from build123d import *

# Parameters (mm, degrees)
CYLINDER_R     = 10
CYLINDER_DEPTH = 2
BOX_W          = 50
BOX_H          = 51
BOX_DEPTH      = 3
BOX001_W       = 50
BOX001_H       = 1
BOX001_DEPTH   = 25
ARRAY_Y_COUNT  = 11
ARRAY_Y_PITCH  = 5


with BuildPart() as cylinder:
    # Cylinder → Cylinder (new body)
    with BuildSketch(Plane.XY):
        Circle(CYLINDER_R)
    extrude(amount=CYLINDER_DEPTH)


with BuildPart() as cube:
    # Box → Box (new body)
    with BuildSketch(Plane(origin=(-25, -25, 0), x_dir=(1, 0, 0), z_dir=(0, 0, 1))):
        with Locations((25, 25.5)):
            Rectangle(BOX_W, BOX_H)
    extrude(amount=BOX_DEPTH)


with BuildPart() as fusion:
    # Box001 → Box001 (new body)
    with BuildSketch(Plane(origin=(-25, -25, 3), x_dir=(1, 0, 0), z_dir=(0, 0, 1))):
        with Locations((25, 0.5)):
            Rectangle(BOX001_W, BOX001_H)
    extrude(amount=BOX001_DEPTH)

    # Array Y: Fusion ×11


with BuildPart() as fusion_1:
    add(fusion.part)
    with Locations(*[(0, i * ARRAY_Y_PITCH, 0) for i in range(1, ARRAY_Y_COUNT)]):
        add(fusion.part)

    # Fusion: union Cylinder, Cube
    add(cylinder.part)
    add(cube.part)


solid = fusion_1.part
Read the model definition and answer for the solid it produces. Units are mm, in the model's axes. Give positions to 0.01 mm unless a question says otherwise; leave off trailing zeros. Write each loop counter-clockwise with the first axis right and the second up, starting at its lowest first coordinate (ties: lowest second). Pieces come first, ordered by that corner, then holes. Notation, with made-up numbers: M -32.75,52.5 L -17.75,52.5 A19 cw -17.75,62.5 Z; hole C 52,47.5 d1. An arc over 180 degrees is marked long. One line per item, written item: value. Start each with the question number.
(1) Determine the mould class of faces 1 (the flat face through (0, -17, 3)), 2 (the flat face through (25, 0.4, 9.8)), 3 (the flat face through (0, -20, 15)), 4 (the flat face through (0, -25, 14)) for opening direction Y: pulls with the +Y half, pulls with the -Y half, needs draft (parallel to the pull), parting line crosses it, or undercut.
(2) Flat-ended cylindrical pins translate along their axes: pin 1 Ø1.5 at (y, z) = (-11.5, 24.5) entering from -X; pin 2 Ø2 at (x, y) = (5, -7.5) entering from +Z. Find the tip coordinate at first contact, or state that the pin passes through.
(3) Find the intervals of material crossed by line 1 (Z direction, x = -21, y = -18.5), in increasing order.
(4) Find section B-B (y = 7.5). Determine the outline of the cut face in (x, z).
(5) Find section A-A (z = 18). Give the number of separate pieces and of enclosed holes in the cut face, plus the area to 3 significant figures.
Results below:
1. face 1: undercut
1. face 2: needs draft
1. face 3: undercut
1. face 4: pulls with the -Y half
2. pin 1: passes through
2. pin 2: stops at z = 3
3. line 1: z = 0 to 3
4. outline: M -25,0 L 25,0 L 25,3 L -25,3 Z
5. separate pieces: 11
5. enclosed holes: 0
5. area: 550 mm^2
